```python
from build123d import *

# Parameters (mm, degrees)
FILLET1_R         = 0.5
DOME1_FACE_RADIUS = 4.5
DOME1_HEIGHT      = 0.5


with BuildPart() as part:
    # Sketch1 → Revolve1 (revolve)
    with BuildSketch(Plane.XY):
        Polygon((0, 0), (5, 0), (5, -40.4), (2.5, -40.4), (2.5, -90.4), (0, -90.4), align=None)
    revolve(axis=Axis((0, -90.4, 0), (0, 1, 0)))

    # Fillet1
    fillet1_edges = [part.edges().sort_by_distance(p)[0] for p in [
        (-5, -40.4, 0),
        (-5, 0, 0),
    ]]
    fillet(fillet1_edges, radius=FILLET1_R)

    # Dome1: a dome of height H over a round flat face of radius A is a cap of a sphere of radius (A * A + H * H) / (2 * H)
    dome1_r = (DOME1_FACE_RADIUS * DOME1_FACE_RADIUS + DOME1_HEIGHT * DOME1_HEIGHT) / (2 * DOME1_HEIGHT)
    dome1_base = Plane((0, 0, 0), z_dir=(0, 1, 0))
    with Locations(dome1_base.offset(DOME1_HEIGHT - dome1_r)):
        dome1_ball = Sphere(dome1_r, mode=Mode.PRIVATE)
    add(split(dome1_ball, bisect_by=dome1_base, keep=Keep.TOP, mode=Mode.PRIVATE))


solid = part.part
```
Here's how the part is built. I have some questions about the finished solid (model axes, mm). A direction names the side the tool comes from. Give positions to 0.01 mm unless a question says otherwise; leave off trailing zeros. Write each loop counter-clockwise with the first axis right and the second up, starting at its lowest first coordinate (ties: lowest second). Pieces come first, ordered by that corner, then holes.
(1) Will these pins go through, and if not, where does the flat tip stop? pin 1 (2 mm diameter, centred on y = -11, z = 1.5, fed in from +X); pin 2 (1 mm diameter, centred on y = -17, z = 3.5, fed in from -X); pin 3 (6 mm diameter, centred on y = -77.5, z = -1.5, fed in from -X); pin 4 (5 mm diameter, centred on x = 2, z = 1, fed in from +Y).
Output values:
pin 1: stops at x = 4.97
pin 2: stops at x = -4
pin 3: stops at x = -2.5
pin 4: stops at y = 0.5
(2) Imagine slicing it at B-B, the plane x = 0. Write out the boundary of the cut face in (y, z), and give its area (3 significant figures).
Output values:
outline: (-90.4, -2.5) - (-40.4, -2.5) - (-40.4, -4.5) arc R0.5 ccw to (-39.9, -5) - (-0.5, -5) arc R0.5 ccw to (0, -4.5) arc R20.5 ccw to (0, 4.5) arc R0.5 ccw to (-0.5, 5) - (-39.9, 5) arc R0.5 ccw to (-40.4, 4.5) - (-40.4, 2.5) - (-90.4, 2.5) - close
area: 657 mm2
(3) Imagine slicing it at C-C, the plane y = -66.5. Write out the boundary of the cut face in (x, z), and give its area (3 significant figures).
Output values:
outline: circle Ø5 at (0, 0)
area: 19.6 mm2
(4) Imagine slicing it at A-A, the plane z = 0. Write out the boundary of the cut face in (x, y), and give its area (3 significant figures).
Output values:
outline: (-5, -39.9) arc R0.5 ccw to (-4.5, -40.4) - (-2.5, -40.4) - (-2.5, -90.4) - (2.5, -90.4) - (2.5, -40.4) - (4.5, -40.4) arc R0.5 ccw to (5, -39.9) - (5, -0.5) arc R0.5 ccw to (4.5, 0) arc R20.5 ccw to (-4.5, 0) arc R0.5 ccw to (-5, -0.5) - close
area: 657 mm2
(5) On a 3-axis mill with a long thin cutter (end or side, diameter ignored), from which of +Z, -Z, +X, -X, +Y, -Y can I reach the whole of each face in a straight line? I mean faces 1 (the face through (-0.54, -65.75, 2.44)), 2 (the face through (-1.08, -20.48, 4.88)). Say none if no direction works.
Output values:
face 1: -Y
face 2: +Y, -Y
(6) Imagine slicing it at D-D, the plane y = -7. Write out the boundary of the cut face in (x, z), and give its area (3 significant figures).
Output values:
outline: circle Ø10 at (0, 0)
area: 78.5 mm2
(7) If I drill on L1, parallel to X at y = -40, z = 0; L2, parallel to X at y = -55, z = 1; L3, parallel to Y at x = 3.5, z = -3.5, over which ranges is the centre line in solid material (lowest first)?
Output values:
L1: x = -4.99 to 4.99
L2: x = -2.29 to 2.29
L3: y = -40.12 to -0.28
